The listing builds one solid part. Answer for the finished solid, in the listing's coordinates (mm). Face numbers are marked on the shaded views. A direction names the side the tool comes from. Coordinates: 2 decimals unless noted, no trailing zeros. Order: outer loops, then holes, each group sorted by start corner. A loop starts at its lowest first (then second) coordinate and runs counter-clockwise, first axis right, second up.
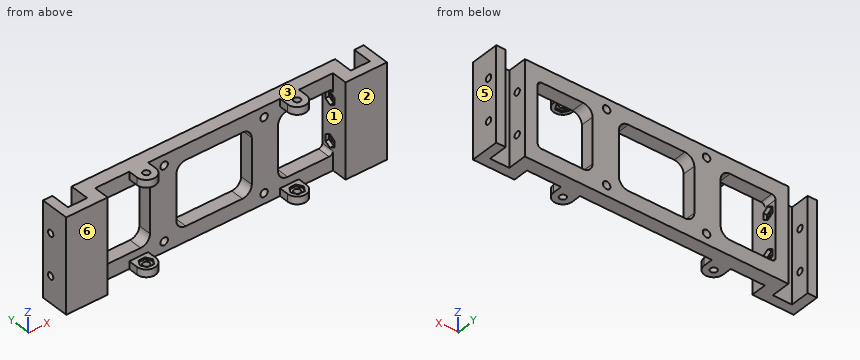
from build123d import *

# Parameters (mm, degrees)
DODANIE_WYCI_GNI_CIE1_DEPTH = 50
SZKIC2_R                    = 2
WYTNIJ_WYCI_GNI_CIE1_DEPTH  = 35
SZKIC3_W                    = 40
SZKIC3_H                    = 34
SZKIC3_W_2                  = 29.1
WYTNIJ_WYCI_GNI_CIE2_DEPTH  = 35
SZKIC4_R                    = 1.75
WYTNIJ_WYCI_GNI_CIE3_DEPTH  = 35
WYTNIJ_WYCI_GNI_CIE4_START  = -22
WYTNIJ_WYCI_GNI_CIE4_DEPTH  = 2
WYTNIJ_WYCI_GNI_CIE5_START  = -148.2
WYTNIJ_WYCI_GNI_CIE5_DEPTH  = 2
SZKIC7_R                    = 1.75
DODANIE_WYCI_GNI_CIE4_DEPTH = 4
WYTNIJ_WYCI_GNI_CIE6_DEPTH  = 1
ZAOKR_GLENIE1_R             = 2
ZAOKR_GLENIE2_R             = 5


with BuildPart() as part:
    # Szkic1 → Dodanie-wyciągnięcie1 (new body)
    with BuildSketch(Plane.XY):
        Polygon((-80.1, -5.1), (-80.1, 5.1), (-85.1, 5.1), (-85.1, -10.1), (-63.1, -10.1), (-63.1, -1.9), (63.1, -1.9), (63.1, -10.1), (85.1, -10.1), (85.1, 5.100203132), (80.100203132, 5.100203132), (80.100203132, -5.100203132), (69.899796868, -5.100203132), (69.899796868, 5.100203132), (-69.9, 5.1), (-69.9, -5.1), align=None)
    extrude(amount=DODANIE_WYCI_GNI_CIE1_DEPTH)

    # Szkic2 → Wytnij-wyciągnięcie1 (cut)
    with BuildSketch(Plane.XZ.offset(10.1)):
        with Locations(Location((-26.5, 44.5, 0), (0, 0, 180))):
            Circle(SZKIC2_R)
        with Locations(Location((-26.5, 5.5, 0), (0, 0, 180))):
            Circle(SZKIC2_R)
        with Locations(Location((26.5, 5.5, 0), (0, 0, 180))):
            Circle(SZKIC2_R)
        with Locations(Location((26.5, 44.5, 0), (0, 0, 180))):
            Circle(SZKIC2_R)
    extrude(amount=-WYTNIJ_WYCI_GNI_CIE1_DEPTH, mode=Mode.SUBTRACT)

    # Szkic3 → Wytnij-wyciągnięcie2 (cut)
    with BuildSketch(Plane.XZ.offset(10.1)):
        with Locations((0, 25)):
            Rectangle(SZKIC3_W, SZKIC3_H)
        with Locations((-48.55, 25)):
            Rectangle(SZKIC3_W_2, SZKIC3_H)
        with Locations((48.55, 25)):
            Rectangle(SZKIC3_W_2, SZKIC3_H)
    extrude(amount=-WYTNIJ_WYCI_GNI_CIE2_DEPTH, mode=Mode.SUBTRACT)

    # Szkic4 → Wytnij-wyciągnięcie3 (cut)
    with BuildSketch(Plane(origin=(85.1, 0, 0), x_dir=(0, 0, -1), z_dir=(1, 0, 0))):
        with Locations((-36, 0.100203132)):
            Circle(SZKIC4_R)
        with Locations((-14, 0.100203132)):
            Circle(SZKIC4_R)
    wytnij_wyci_gni_cie3 = extrude(amount=-WYTNIJ_WYCI_GNI_CIE3_DEPTH, mode=Mode.SUBTRACT)

    # Szkic5 → Wytnij-wyciągnięcie4 (cut)
    with BuildSketch(Plane(origin=(85.1, 0, 0), x_dir=(0, 0, -1), z_dir=(1, 0, 0)).offset(WYTNIJ_WYCI_GNI_CIE4_START)):
        Polygon((-34.267949192, 3.100203132), (-37.732050808, 3.100203132), (-39.464101615, 0.100203132), (-37.732050808, -2.899796868), (-34.267949192, -2.899796868), (-32.535898385, 0.100203132), align=None)
        Polygon((-12.267949192, 3.100203132), (-15.732050808, 3.100203132), (-17.464101615, 0.100203132), (-15.732050808, -2.899796868), (-12.267949192, -2.899796868), (-10.535898385, 0.100203132), align=None)
    extrude(amount=WYTNIJ_WYCI_GNI_CIE4_DEPTH, mode=Mode.SUBTRACT)

    # Lustro1: Wytnij-wyciągnięcie3 across plane
    add(wytnij_wyci_gni_cie3.mirror(Plane(origin=(0, 0, 0), x_dir=(0, 0, 1), z_dir=(1, 0, 0))), mode=Mode.SUBTRACT)

    # Szkic5<2> → Wytnij-wyciągnięcie5 (cut)
    with BuildSketch(Plane(origin=(85.1, 0, 0), x_dir=(0, 0, -1), z_dir=(1, 0, 0)).offset(WYTNIJ_WYCI_GNI_CIE5_START)):
        Polygon((-34.267949192, 3.100203132), (-37.732050808, 3.100203132), (-39.464101615, 0.100203132), (-37.732050808, -2.899796868), (-34.267949192, -2.899796868), (-32.535898385, 0.100203132), align=None)
        Polygon((-12.267949192, 3.100203132), (-15.732050808, 3.100203132), (-17.464101615, 0.100203132), (-15.732050808, -2.899796868), (-12.267949192, -2.899796868), (-10.535898385, 0.100203132), align=None)
    extrude(amount=-WYTNIJ_WYCI_GNI_CIE5_DEPTH, mode=Mode.SUBTRACT)

    # Szkic7 → Dodanie-wyciągnięcie4 (add)
    # profile 1 of 2: a face of its own
    with BuildSketch(Plane.XY.offset(50)):
        with BuildLine():
            Line((-34.999927458, -1.9), (-44.999927458, -1.9))
            Line((-44.999927458, -1.9), (-44.999927458, -6.9))
            ThreePointArc((-44.999927458, -6.9), (-39.999927458, -11.9), (-34.999927458, -6.9))
            Line((-34.999927458, -6.9), (-34.999927458, -1.9))
        make_face()
        with Locations((-39.999927458, -6.9)):
            Circle(SZKIC7_R, mode=Mode.SUBTRACT)
    # profile 2 of 2: a face of its own
    with BuildSketch(Plane.XY.offset(50)):
        with BuildLine():
            Line((35.000072542, -1.9), (35.000072542, -6.9))
            ThreePointArc((35.000072542, -6.9), (40.000072542, -11.9), (45.000072542, -6.9))
            Line((45.000072542, -6.9), (45.000072542, -1.9))
            Line((45.000072542, -1.9), (35.000072542, -1.9))
        make_face()
        with Locations((40.000072542, -6.9)):
            Circle(SZKIC7_R, mode=Mode.SUBTRACT)
    dodanie_wyci_gni_cie4 = extrude(amount=-DODANIE_WYCI_GNI_CIE4_DEPTH)

    # Szkic8 → Wytnij-wyciągnięcie6 (cut)
    with BuildSketch(Plane(origin=(0, 0, 46), x_dir=(-1, 0, 0), z_dir=(0, 0, -1))):
        Polygon((43.464029073, -6.9), (41.731978266, -3.9), (38.26787665, -3.9), (36.535825843, -6.9), (38.26787665, -9.9), (41.731978266, -9.9), align=None)
        Polygon((-36.535970927, -6.9), (-38.268021734, -3.9), (-41.73212335, -3.9), (-43.464174157, -6.9), (-41.73212335, -9.9), (-38.268021734, -9.9), align=None)
    wytnij_wyci_gni_cie6 = extrude(amount=-WYTNIJ_WYCI_GNI_CIE6_DEPTH, mode=Mode.SUBTRACT)

    # Lustro3: Dodanie-wyciągnięcie4, Wytnij-wyciągnięcie6 across plane
    add(dodanie_wyci_gni_cie4.mirror(Plane(origin=(0, 0, 25), x_dir=(1, 0, 0), z_dir=(0, 0, -1))))
    add(wytnij_wyci_gni_cie6.mirror(Plane(origin=(0, 0, 25), x_dir=(1, 0, 0), z_dir=(0, 0, -1))), mode=Mode.SUBTRACT)

    # Zaokrąglenie1
    zaokr_glenie1_edges = [part.edges().sort_by_distance(p)[0] for p in [
        (-63.1, 1.60000494, 8),
        (-63.1, 1.60000494, 42),
        (63.1, 1.600096626, 42),
        (63.1, 1.600096626, 8),
    ]]
    fillet(zaokr_glenie1_edges, radius=ZAOKR_GLENIE1_R)

    # Zaokrąglenie2
    zaokr_glenie2_edges = [part.edges().sort_by_distance(p)[0] for p in [
        (-34, 1.600026082, 8),
        (20, 1.600065313, 42),
        (20, 1.600065313, 8),
        (-20, 1.600036253, 8),
        (-20, 1.600036253, 42),
        (34, 1.600075485, 8),
        (34, 1.600075485, 42),
        (-34, 1.600026082, 42),
    ]]
    fillet(zaokr_glenie2_edges, radius=ZAOKR_GLENIE2_R)


solid = part.part
1) Determine the mould class of the marked faces 4, 5 and 6 for opening direction X: released by +X, released by -X, zero draft, split by the parting line, or undercut.
2) Each of these flat-tipped pins is pushed along its axis until it touches: P1, Ø1.6, axis at x = 64, z = 36, coming from the -Y side; P2, Ø2.5, axis at x = -26.5, z = 44.5, coming from the -Y side; P3, Ø15, axis at x = 25, z = 13, coming from the -Y side. Where does it stop, or does it pass through?
3) Section B-B (x = 26.5) is taken. Give the vertices of the cut face in (y, z), then the cut area to 3 significant figures.
4) Section C-C (z = 29) is taken. Give the vertices of the cut face in (x, y).
5) A tool of negligible diameter and unlimited length cuts with its end or side. For the marked faces 1, 2 and 3, from which of +Z, -Z, +X, -X, +Y, -Y can it reach the whole face along a straight path? Write none if from no direction.
6) Section A-A (z = 44.5) is taken. Give the vertices of the cut face in (x, y), then the cut area to 3 significant figures.
7) Consider L1, parallel to X at y = 0, z = 5.5; L2, parallel to X at y = 0, z = 20.5; L3, parallel to X at y = -2, z = 27. Determine where each line is inside the solid, lowest interval first.
Filled sheet:
1. face 4: undercut
1. face 5: released by +X
1. face 6: zero draft
2. P1: stops at y = -10.1
2. P2: passes through
2. P3: stops at y = -1.9
3. outline: (-1.9, 0) - (5.1, 0) - (5.1, 3.5) - (-1.9, 3.5) - close; (-1.9, 7.5) - (5.1, 7.5) - (5.1, 42.5) - (-1.9, 42.5) - close; (-1.9, 46.5) - (5.1, 46.5) - (5.1, 50) - (-1.9, 50) - close
3. area: 294 mm2
4. outline: (-85.1, -10.1) - (-63.1, -10.1) - (-63.1, 5.1) - (-69.9, 5.1) - (-69.9, -5.1) - (-80.1, -5.1) - (-80.1, 5.1) - (-85.1, 5.1) - close; (-34, -1.9) - (-20, -1.9) - (-20, 5.1) - (-34, 5.1) - close; (20, -1.9) - (34, -1.9) - (34, 5.1) - (20, 5.1) - close; (63.1, -10.1) - (85.1, -10.1) - (85.1, 5.1) - (80.1, 5.1) - (80.1, -5.1) - (69.9, -5.1) - (69.9, 5.1) - (63.1, 5.1) - close
5. face 1: -Y
5. face 2: +Z, -Z, +X, -Y
5. face 3: +Z, +X, -X, +Y, -Y
6. outline: (-85.1, -10.1) - (-63.1, -10.1) - (-63.1, -1.9) - (-28.5, -1.9) - (-28.5, 5.1) - (-69.9, 5.1) - (-69.9, -5.1) - (-80.1, -5.1) - (-80.1, 5.1) - (-85.1, 5.1) - close; (-24.5, -1.9) - (24.5, -1.9) - (24.5, 5.1) - (-24.5, 5.1) - close; (28.5, -1.9) - (63.1, -1.9) - (63.1, -10.1) - (85.1, -10.1) - (85.1, 5.1) - (80.1, 5.1) - (80.1, -5.1) - (69.9, -5.1) - (69.9, 5.1) - (28.5, 5.1) - close
6. area: 1,290 mm2
7. L1: x = -85.1 to -80.1, -69.9 to -28.5, -24.5 to 24.5, 28.5 to 69.9, 80.1 to 85.1
7. L2: x = -85.1 to -80.1, -69.9 to -63.1, -34 to -20, 20 to 34, 63.1 to 69.9, 80.1 to 85.1
7. L3: x = -85.1 to -80.1, -69.9 to -63.1, 63.1 to 69.9, 80.1 to 85.1
